Read the model definition and answer for the solid it produces. Units are mm, in the model's axes. Face numbers are marked on the shaded views. A direction names the side the tool comes from. Give positions to 0.01 mm unless a question says otherwise; leave off trailing zeros. Loops run counter-clockwise (first coordinate to the right, second up) from the corner with the lowest first, then second, coordinate; pieces in that order, holes last.
(1) Find section B-B, the plane z = -5.5. Write down the section's boundary in (x, y), then the cut area to 3 significant figures.
(2) Find section A-A, the plane y = 0. Write down the section's boundary in (x, z).
(3) Which of the six approach directions +Z, -Z, +X, -X, +Y, -Y give full straight-line access (tool end or side, diameter ignored) to the marked faces 1 and 2?
(4) Find section C-C, the plane x = 84.5. Write down the section's boundary in (y, z).
(5) Each of these flat-tipped pins is pushed along its axis until it touches: P1, Ø0.8, axis at x = 87.5, y = 7, coming from the +Z side; P2, Ø8, axis at x = 71, y = -5.5, coming from the -Z side; P3, Ø12, axis at x = 89, z = -3.5, coming from the +Y side. Where does it stop, or does it pass through?
(6) Straight lines are drawn through the part: probe 1 along X at (y, z) = (-7.25, -5.25); probe 2 along Z at (x, y) = (82, 0); probe 3 along X at (y, z) = (6.5, -1.5). For each, find the intervals that lie inside material, in ascending order.
(7) Find section D-D, the plane x = 29. Write down the section's boundary in (y, z), then the cut area to 3 significant figures.
```python
from build123d import *

# Parameters (mm, degrees)
ESBO_O2_W                  = 1
ESBO_O2_H                  = 0.4
CORTE_EXTRUS_O1_DEPTH      = 104.166128162
CORTE_EXTRUS_O1_DEPTH_BACK = 3
CORTE_EXTRUS_O7_DEPTH      = 3
ESBO_O6_W                  = 17
ESBO_O6_H                  = 0.05


with BuildPart() as part:
    # Esboço1 → Revolução1 (revolve)
    with BuildSketch(Plane.XY):
        Polygon((0, 0), (0, 8.5), (25, 8.5), (25, 10), (36, 10), (36, 8.5), (101, 8.5), (101, 0), align=None)
    revolve(axis=Axis((101, 0, 0), (-1, 0, 0)))

    # Esboço2 → Corte-Revolução1 (revolve, cut)
    with BuildSketch(Plane.XY):
        with Locations((98.5, 8.3)):
            Rectangle(ESBO_O2_W, ESBO_O2_H)
    revolve(axis=Axis((0, 0, 0), (1, 0, 0)), mode=Mode.SUBTRACT)

    # Esboço3 → Corte-extrusão1 (cut, two sides: drawn at the far end of the back side and taken through both)
    with BuildSketch(Plane(origin=(0, 8.5, 0), x_dir=(1, 0, 0), z_dir=(0, 1, 0)).offset(-CORTE_EXTRUS_O1_DEPTH_BACK)):
        with BuildLine():
            Line((75, -2.5), (105, -2.5))
            ThreePointArc((105, -2.5), (107.5, 0), (105, 2.5))
            Line((105, 2.5), (75, 2.5))
            ThreePointArc((75, 2.5), (72.5, 0), (75, -2.5))
        make_face()
    extrude(amount=CORTE_EXTRUS_O1_DEPTH + CORTE_EXTRUS_O1_DEPTH_BACK, mode=Mode.SUBTRACT)

    # Esboço5 → Corte-extrusão7 (cut)
    with BuildSketch(Plane(origin=(0, 8.5, 0), x_dir=(-1, 0, 0), z_dir=(0, 1, 0))):
        with BuildLine():
            Line((-2.51, 2.5), (-22.51, 2.5))
            ThreePointArc((-22.51, 2.5), (-25.01, 0), (-22.51, -2.5))
            Line((-22.51, -2.5), (-2.51, -2.5))
            ThreePointArc((-2.51, -2.5), (-0.01, 0), (-2.51, 2.5))
        make_face()
    extrude(amount=-CORTE_EXTRUS_O7_DEPTH, mode=Mode.SUBTRACT)

    # Esboço6 → Corte-Revolução2 (revolve, cut)
    with BuildSketch(Plane(origin=(0, 0, 0), x_dir=(1, 0, 0), z_dir=(0, 1, 0)), mode=Mode.PRIVATE) as corte_revolu_o2_sk:
        with Locations((54.5, 8.475)):
            Rectangle(ESBO_O6_W, ESBO_O6_H)
    revolve(corte_revolu_o2_sk.sketch.rotate(Axis((48.876141687, 0, 0), (1, 0, 0)), 90), axis=Axis((48.876141687, 0, 0), (1, 0, 0)), mode=Mode.SUBTRACT)


solid = part.part
```
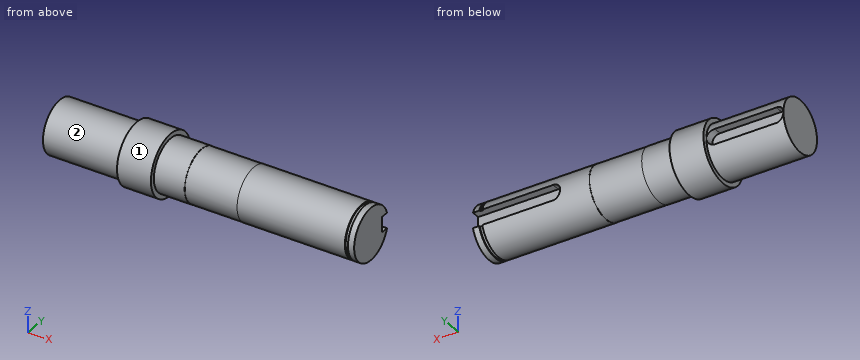
Entries:
1. outline: (0, -6.48) - (25, -6.48) - (25, -8.35) - (36, -8.35) - (36, -6.48) - (46, -6.48) - (46, -6.42) - (63, -6.42) - (63, -6.48) - (98, -6.48) - (98, -5.95) - (99, -5.95) - (99, -6.48) - (101, -6.48) - (101, 6.48) - (99, 6.48) - (99, 5.95) - (98, 5.95) - (98, 6.48) - (63, 6.48) - (63, 6.42) - (46, 6.42) - (46, 6.48) - (36, 6.48) - (36, 8.35) - (25, 8.35) - (25, 6.48) - (0, 6.48) - close
1. area: 1,350 mm2
2. outline: (0, -8.5) - (25, -8.5) - (25, -10) - (36, -10) - (36, -8.5) - (46, -8.5) - (46, -8.45) - (63, -8.45) - (63, -8.5) - (98, -8.5) - (98, -8.1) - (99, -8.1) - (99, -8.5) - (101, -8.5) - (101, 8.5) - (99, 8.5) - (99, 8.1) - (98, 8.1) - (98, 8.5) - (63, 8.5) - (63, 8.45) - (46, 8.45) - (46, 8.5) - (36, 8.5) - (36, 10) - (25, 10) - (25, 8.5) - (0, 8.5) - close
3. face 1: +X, -X
3. face 2: -X
4. outline: (5.5, -2.5) - (5.5, 2.5) - (8.12, 2.5) arc R8.5 ccw (long way) to (8.12, -2.5) - close
5. P1: stops at z = 5.36
5. P2: stops at z = -8.37
5. P3: stops at y = 8.12
6. probe 1: x = 25 to 36
6. probe 2: z = -8.5 to 8.5
6. probe 3: x = 0 to 0.51, 24.51 to 73
7. outline: circle Ø20 at (0, 0)
7. area: 314 mm2
